Autodesk Inventor part; units mm, degrees
ref_plane "YZ Plane" through (0, 0, 0) normal (1, 0, 0) x (0, 1, 0)
ref_plane "XZ Plane" through (0, 0, 0) normal (0, 1, 0) x (-1, 0, 0)
ref_plane "XY Plane" through (0, 0, 0) normal (0, 0, 1) x (1, 0, 0)
sketch "Sketch1" plane through (0, 0, 0) normal (0, 0, 1) x (1, 0, 0)
  line L0 (0, 0) -> (152.4, 0)
  line L1 (152.4, 0) -> (152.4, 99.06)
  line L2 (152.4, 99.06) -> (0, 99.06)
  line L3 (0, 99.06) -> (0, 0)
  dimension "d0" = 152.4
  dimension "d1" = 99.06
extrude "Extrusion1" add sketch "Sketch1" along normal blind 1.8542
sketch "Sketch2" plane through (0, 0, 1.8542) normal (0, 0, 1) x (1, 0, 0)
  line L0 (0, 99.06) -> (0, 0)
  line L1 (152.4, 99.06) -> (0, 99.06)
  line L2 (152.4, 0) -> (152.4, 99.06)
  point P0 (14.1478, 21.4884)
  point P1 (14.1478, 5.4884)
  point P2 (138.2522, 21.4884)
  point P3 (138.2522, 5.4884)
  dimension "d4" = 16
  dimension "d5" = 14.1478
  dimension "d6" = 14.1478
  dimension "d7" = 77.5716
  dimension "d8" = 16
  dimension "d9" = 14.1478
  dimension "d10" = 14.1478
  dimension "d11" = 77.5716
hole "Hole1" at (14.1478, 21.4884, 1.8542) at (14.1478, 5.4884, 1.8542) at (138.2522, 21.4884, 1.8542) at (138.2522, 5.4884, 1.8542) direction (0, 0, -1) diameter 3.81 depth 10.9728 tip angle 118
properties part number "PaddleCollection2.1Backing" material "Polycarbonate, Clear"
Can you work these out from the model? Positions are in its coordinate system, mm. Give positions to 0.01 mm unless a question says otherwise; leave off trailing zeros. Order: outer loops, then holes, each group sorted by start corner. A loop starts at its lowest first (then second) coordinate and runs counter-clockwise, first axis right, second up. Notation, with made-up numbers: M 66,27.25 L 114,27.25 A11 ccw 114,39.25 Z; hole C -16,44.25 d1. An arc over 180 degrees is marked long. One line per item, written item: value.
1) For P1, Ø2.5, axis at x = 14.15, y = 5.49, coming from the -Z side, with a flat end and sliding along its axis, tell me the tip position at first contact or that it passes through.
Answer sheet:
P1: passes through
2) We'd pull the mould along X, two halves only. Please class faces 1 (the face through (13.58, 19.67, 0.91)), 2 (the face through (75, 50, 0)), 3 (the face through (139.942, 20.609, 0.914)): released by +X, released by -X, zero draft, split by the parting line, or undercut.
Answer sheet:
face 1: undercut
face 2: zero draft
face 3: undercut
3) I want a section at A-A, the plane y = 21.5. List the corners of the cut face in (x, z) for me, plus the area to 3 significant figures.
Answer sheet:
outline: M 0,0 L 12.24,0 L 12.24,1.85 L 0,1.85 Z; M 16.05,0 L 136.35,0 L 136.35,1.85 L 16.05,1.85 Z; M 140.16,0 L 152.4,0 L 152.4,1.85 L 140.16,1.85 Z
area: 268 mm^2
